Design review of the part built by this model. Coordinates are the model's own, in mm. A direction names the side the tool comes from. Coordinates: 2 decimals unless noted, no trailing zeros. Write each loop counter-clockwise with the first axis right and the second up, starting at its lowest first coordinate (ties: lowest second). Pieces come first, ordered by that corner, then holes.
Q1. For pin 1 Ø9.5 at (x, z) = (-27.5, 17.5) entering from +Y; pin 2 Ø2.5 at (y, z) = (4, -38) entering from -X; pin 3 Ø1.8 at (y, z) = (3.5, -29) entering from +X, all flat-tipped, find the tip position at first contact; note any pin that passes through.
Q2. For L1, parallel to X at y = 4, z = 0.5; L2, parallel to Z at x = 0, y = 3.55; L3, parallel to X at y = 3.9, z = -9, list the stretches that pass through material, from the lowest coordinate up.
Q3. For faces 1 (the flat face through (21, 4.8, 7)), 2 (the flat face through (-0.865, 4, -33)), list the 3-axis set-ups (+Z, -Z, +X, -X, +Y, -Y) from which the entire face can be reached by the end or side of a thin tool; tool diameter is ignored.
Q4. The part is to be moulded in two halves that separate along Z. For faces 3 (the flat face through (15.2, 3.63, 29.57)), 4 (the flat face through (21, 0, 10)), 5 (the cylindrical face through (-10.536, 1.232, -47.444)), say which applies: released by +Z, released by -Z, zero draft, split by the parting line, or undercut.
Q5. Take a section at D-D, the plane x = 29.5. Write out the cut boundary in (y, z).
Q6. Take a section at B-B, the plane x = 40. Write out the cut boundary in (y, z), plus the area to 3 significant figures.
Q7. Take a section at C-C, the plane y = 0.8. Write out the cut boundary in (x, z).
Q8. Take a section at A-A, the plane z = 31. Write out the cut boundary in (x, y), plus the area to 3 significant figures.
Autodesk Fusion 360 part; units mm, degrees
sketch "Sketch1" plane through (0, 0, 0) normal (0, 1, 0) x (1, 0, 0)
  circle A0 centre (0, 0) radius 48.6
  circle A1 centre (0, 0) radius 21
  dimension "d1" = 97.2
  dimension "d7" = 42
extrude "Extrude1" add sketch "Sketch1" along normal blind 2.5
sketch "support_ribs" plane through (0, 2.5, 0) normal (0, 1, 0) x (-1, 0, 0)
  circle A0 centre (0, 0) radius 21
  circle A1 centre (0, 0) radius 48.6
  circle A2 centre (0, 0) radius 45.8
  circle A3 centre (0, 0) radius 44
  circle A4 centre (0, 0) radius 21
  circle A5 centre (0, 0) radius 22.8
  line L0 (-0.9352, -21.9) -> (0.8648, -21.9)
  line L1 (0.8648, -21.9) -> (0.8648, -44.9)
  line L2 (0.8648, -44.9) -> (-0.9352, -44.9)
  line L3 (-0.9352, -44.9) -> (-0.9352, -21.9)
  line L4 (-0.9352, -21.9) -> (0.8648, -44.9) construction
  line L5 (0.8648, -21.9) -> (-0.9352, -44.9) construction
  dimension "d12" = 91.6
  dimension "d13" = 88
  dimension "d14" = 42
  dimension "d15" = 45.6
  dimension "d16" = 33.4
  dimension "d17" = 1.8
  dimension "d18" = 23
extrude "Extrude2" add sketch "support_ribs" along normal blind 2.3 contours A2 | A3 L1 L2 L3 | A5 L0 L1 L3 | A5 L0 L1 L3
extrude "Extrude3" add sketch "support_ribs" along normal blind 2.3 contours A3 A5 L1 L3 picked at (0.6649, -29.8579)
pattern_circular "C-Pattern1" count 7 over 360 about axis through (0, 1.75, 0) along (0, 1, 0) of "Extrude3"
equation "d1 = insert_dia"
equation "insert_dia = 97.2 mm"
equation "bit_dia = 30 mm"
equation "bit_clearance = 6 mm"
equation "insert_thick = 2.5 mm"
equation "support_rib_height = 2.3 mm"
equation "d7 = bit_dia + bit_clearance * 2"
equation "d8 = insert_thick"
equation "insert_lip = 2.8 mm"
equation "support_rib_width = 1.8 mm"
equation "d12 = insert_dia - 2 * insert_lip"
equation "d13 = insert_dia - 2 * insert_lip - support_rib_width * 2"
equation "d14 = bit_dia + 2 * bit_clearance"
equation "d15 = bit_dia + 2 * bit_clearance + 2 * support_rib_width"
equation "d16 = Linear Dimension-2"
equation "d17 = support_rib_width"
equation "d18 = insert_dia / 2 - insert_lip - bit_dia / 2 - bit_clearance - support_rib_width"
equation "d19 = support_rib_height"
equation "d21 = support_rib_height"
Responses:
1. pin 1: stops at y = 2.5
1. pin 2: stops at x = -27.33
1. pin 3: stops at x = 36.17
2. L1: x = -45.8 to -44, -22.79 to -20.99, 20.99 to 22.79, 44 to 45.8
2. L2: z = -45.8 to -21, 21 to 22.8, 44 to 45.8
2. L3: x = -44.91 to -43.07, -20.95 to -18.97, 18.97 to 20.95, 43.07 to 44.91
3. face 1: +Z, -Z, +X, -X, +Y
3. face 2: +Y
4. face 3: undercut
4. face 4: zero draft
4. face 5: split by the parting line
5. outline: (0, -38.62) - (2.5, -38.62) - (2.5, -35.03) - (4.8, -35.03) - (4.8, -32.65) - (2.5, -32.65) - (2.5, -24.63) - (4.8, -24.63) - (4.8, -22.33) - (2.5, -22.33) - (2.5, 5.85) - (4.8, 5.85) - (4.8, 7.69) - (2.5, 7.69) - (2.5, 32.65) - (4.8, 32.65) - (4.8, 35.03) - (2.5, 35.03) - (2.5, 38.62) - (0, 38.62) - close
6. outline: (0, -27.6) - (2.5, -27.6) - (2.5, -22.31) - (4.8, -22.31) - (4.8, -18.33) - (2.5, -18.33) - (2.5, 8.24) - (4.8, 8.24) - (4.8, 10.09) - (2.5, 10.09) - (2.5, 18.33) - (4.8, 18.33) - (4.8, 22.31) - (2.5, 22.31) - (2.5, 27.6) - (0, 27.6) - close
6. area: 161 mm2
7. outline: circle Ø97.2 at (0, 0); hole circle Ø42 at (0, 0)
8. outline: (-37.43, 0) - (37.43, 0) - (37.43, 2.5) - (33.71, 2.5) - (33.71, 4.8) - (31.22, 4.8) - (31.22, 2.5) - (15.89, 2.5) - (15.89, 4.8) - (13.89, 4.8) - (13.89, 2.5) - (-13.97, 2.5) - (-13.97, 4.8) - (-15.97, 4.8) - (-15.97, 2.5) - (-31.22, 2.5) - (-31.22, 4.8) - (-33.71, 4.8) - (-33.71, 2.5) - (-37.43, 2.5) - close
8. area: 208 mm2
